Answer from the drawing. Dimensions are ordinates in mm from the lowest x, y and z of the part. A direction names the side the tool comes from. Round coordinates to 2 decimals unless told otherwise and drop trailing zeros. Loops run counter-clockwise (first coordinate to the right, second up) from the corner with the lowest first, then second, coordinate; pieces in that order, holes last.
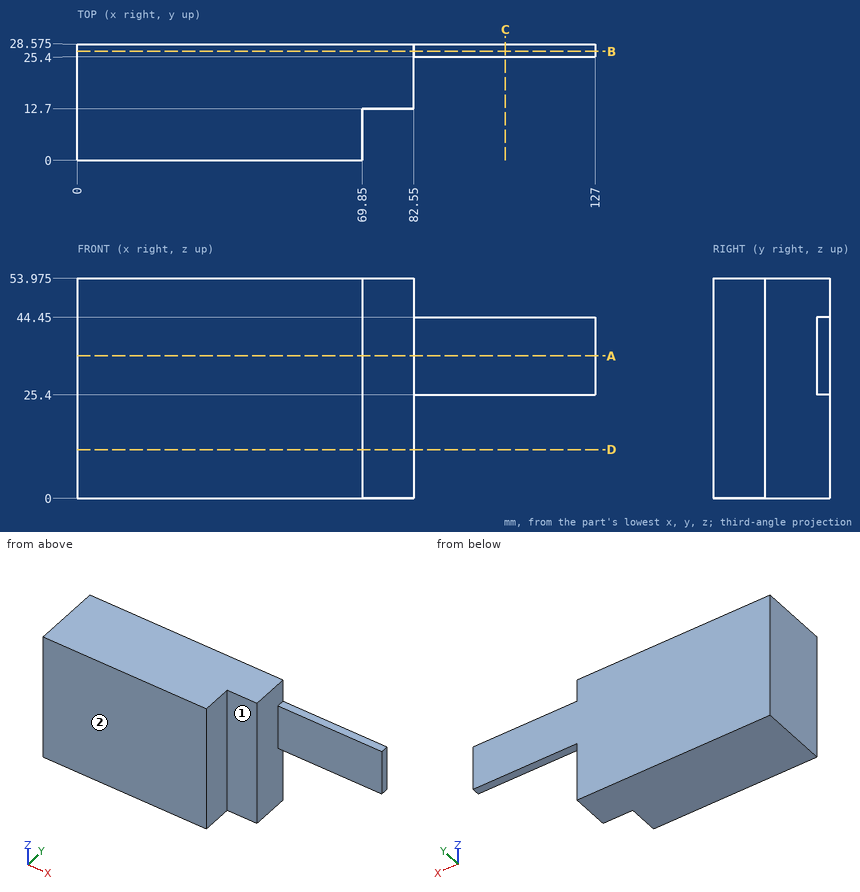
1. Find section B-B (y = 26.75). Write down the section's boundary in (x, z) (3 decimals).
Answer key:
outline: (0, 0) - (82.55, 0) - (82.55, 25.4) - (127, 25.4) - (127, 44.45) - (82.55, 44.45) - (82.55, 53.975) - (0, 53.975) - close
2. Find section C-C (x = 105). Write down the section's boundary in (y, z) (3 decimals).
Answer key:
outline: (25.4, 25.4) - (28.575, 25.4) - (28.575, 44.45) - (25.4, 44.45) - close
3. Given pin 1 (4 mm diameter, centred on x = 104, z = 34, fed in from -Y); pin 2 (2.5 mm diameter, centred on x = 109, y = 27.5, fed in from +Z); pin 3 (1 mm diameter, centred on x = 115.5, y = 26.5, fed in from -Z), each flat-ended and moving along its own axis, determine where each tip first touches the part or whether it passes through.
Answer key:
pin 1: stops at y = 25.4
pin 2: stops at z = 44.45
pin 3: stops at z = 25.4
4. Which of the six approach directions +Z, -Z, +X, -X, +Y, -Y give full straight-line access (tool end or side, diameter ignored) to the marked faces 1 and 2?
Answer key:
face 1: +Z, -Z, +X, -Y
face 2: +Z, -Z, +X, -X, -Y
5. Find section A-A (z = 35). Write down the section's boundary in (x, y) (3 decimals), then the cut area to 3 significant figures.
Answer key:
outline: (0, 0) - (69.85, 0) - (69.85, 12.7) - (82.55, 12.7) - (82.55, 25.4) - (127, 25.4) - (127, 28.575) - (0, 28.575) - close
area: 2,340 mm2
6. Consider probe 1 along X at (y, z) = (14.5, 29.5); probe 2 along Y at (x, z) = (82.5, 9.5) (3 decimals); probe 3 along Y at (x, z) = (118, 39.5) (3 decimals). Determine where each line is inside the solid, lowest interval first.
Answer key:
probe 1: x = 0 to 82.55
probe 2: y = 12.7 to 28.575
probe 3: y = 25.4 to 28.575
7. Find section D-D (z = 12). Write down the section's boundary in (x, y) (3 decimals).
Answer key:
outline: (0, 0) - (69.85, 0) - (69.85, 12.7) - (82.55, 12.7) - (82.55, 28.575) - (0, 28.575) - close
